Autodesk Inventor part; units mm, degrees
ref_plane "YZ Plane" through (0, 0, 0) normal (1, 0, 0) x (0, 1, 0)
ref_plane "XZ Plane" through (0, 0, 0) normal (0, 1, 0) x (-1, 0, 0)
ref_plane "XY Plane" through (0, 0, 0) normal (0, 0, 1) x (1, 0, 0)
sketch "Schizzo1" plane through (0, 0, 0) normal (0, 0, 1) x (1, 0, 0)
  line L0 (-50, 25) -> (50, 25)
  line L1 (50, 25) -> (50, -25)
  line L2 (50, -25) -> (-50, -25)
  line L3 (-50, -25) -> (-50, 25)
  line L4 (-50, 25) -> (50, -25) construction
  line L5 (50, 25) -> (-50, -25) construction
  point P0 (0, 0)
  dimension "d0" = 100
  dimension "d1" = 50
extrude "Estrusione1" add sketch "Schizzo1" along normal blind 8
fillet "Raccordo1" radius 2 4 edges at (-50, 25, 4) (50, 25, 4) (50, -25, 4) (-50, -25, 4)
sketch "Schizzo2" plane through (0, 0, 8) normal (0, 0, 1) x (1, 0, 0)
  circle A0 centre (-40, -19.5) radius 2.067
  line L0 (-48, -25) -> (48, -25)
  line L1 (-50, 23) -> (-50, -23)
  line L2 (50, -23) -> (50, 23)
  point P0 (0, 0)
  point P1 (-40, 8.5)
  point P2 (40, 8.5)
  point P3 (40, -19.5)
  dimension "d13" = 28
  dimension "d16" = 5.5
  dimension "d17" = 10
  dimension "d18" = 10
hole "Foro1" at (-40, -19.5, 8) at (-40, 8.5, 8) at (40, 8.5, 8) at (40, -19.5, 8) direction (0, 0, -1) diameter 5.5 end through all
properties part number "Piastra collegamento asse - pistone"
Could you check a few things on this model? Use its own coordinates, in mm. Give positions to 0.01 mm unless a question says otherwise; leave off trailing zeros. Write each loop counter-clockwise with the first axis right and the second up, starting at its lowest first coordinate (ties: lowest second). Pieces come first, ordered by that corner, then holes. Notation, with made-up numbers: (30.5, 14.5) -> (69.5, 14.5) arc R22 ccw to (69.5, 33.5) -> close; hole circle Ø7 at (42.5, -4.75). An arc over 180 degrees is marked (long way). Write each question's results on one line, items separated by ' | '. Start each with the question number.
Q1. Suppose I cut it at B-B, the plane y = 8.5. List the corners of the cut face in (x, z) for me.
Q2. Suppose I cut it at C-C, the plane z = 6.5. List the corners of the cut face in (x, y) for me.
Q3. I need wall thicknesses on probe 1 along Y at (x, z) = (-40, 4); probe 2 along X at (y, z) = (8.5, 5.5); probe 3 along X at (y, z) = (7, 4). Which ranges of each line are inside material? Lowest first, please.
Q4. Suppose I cut it at A-A, the plane x = -40. List the corners of the cut face in (y, z) for me.
Q5. I'm going to push a flat-ended pin straight in: pin 1 Ø6.5 at (x, y) = (-40, 8.5) entering from +Z. Where does the tip first touch, or does it pass through?
Q6. We'd pull the mould along Y, two halves only. Please class faces 1 (the face through (-42.727, 8.858, 3.944)), 2 (the face through (1, -25, 4)), 3 (the face through (-1, 25, 4)): +Y half, -Y half, draft (parallel to the pull), parting line (faces both ways), or undercut.
Outcome:
1) outline: (-50, 0) -> (-42.75, 0) -> (-42.75, 8) -> (-50, 8) -> close; (-37.25, 0) -> (37.25, 0) -> (37.25, 8) -> (-37.25, 8) -> close; (42.75, 0) -> (50, 0) -> (50, 8) -> (42.75, 8) -> close
2) outline: (-50, -23) arc R2 ccw to (-48, -25) -> (48, -25) arc R2 ccw to (50, -23) -> (50, 23) arc R2 ccw to (48, 25) -> (-48, 25) arc R2 ccw to (-50, 23) -> close; hole circle Ø5.5 at (-40, -19.5); hole circle Ø5.5 at (-40, 8.5); hole circle Ø5.5 at (40, -19.5); hole circle Ø5.5 at (40, 8.5)
3) probe 1: -25 to -22.25, -16.75 to 5.75, 11.25 to 25 | probe 2: -50 to -42.75, -37.25 to 37.25, 42.75 to 50 | probe 3: -50 to -42.3, -37.7 to 37.7, 42.3 to 50
4) outline: (-25, 0) -> (-22.25, 0) -> (-22.25, 8) -> (-25, 8) -> close; (-16.75, 0) -> (5.75, 0) -> (5.75, 8) -> (-16.75, 8) -> close; (11.25, 0) -> (25, 0) -> (25, 8) -> (11.25, 8) -> close
5) pin 1: z = 8
6) face 1: undercut | face 2: -Y half | face 3: +Y half
